Design review of the part shown in the three views and the two pictorial views. Dimensions are in mm from the part's minimum x, y and z. A direction names the side the tool comes from. Round coordinates to 2 decimals unless told otherwise and drop trailing zeros. Order: outer loops, then holes, each group sorted by start corner. A loop starts at its lowest first (then second) coordinate and runs counter-clockwise, first axis right, second up.
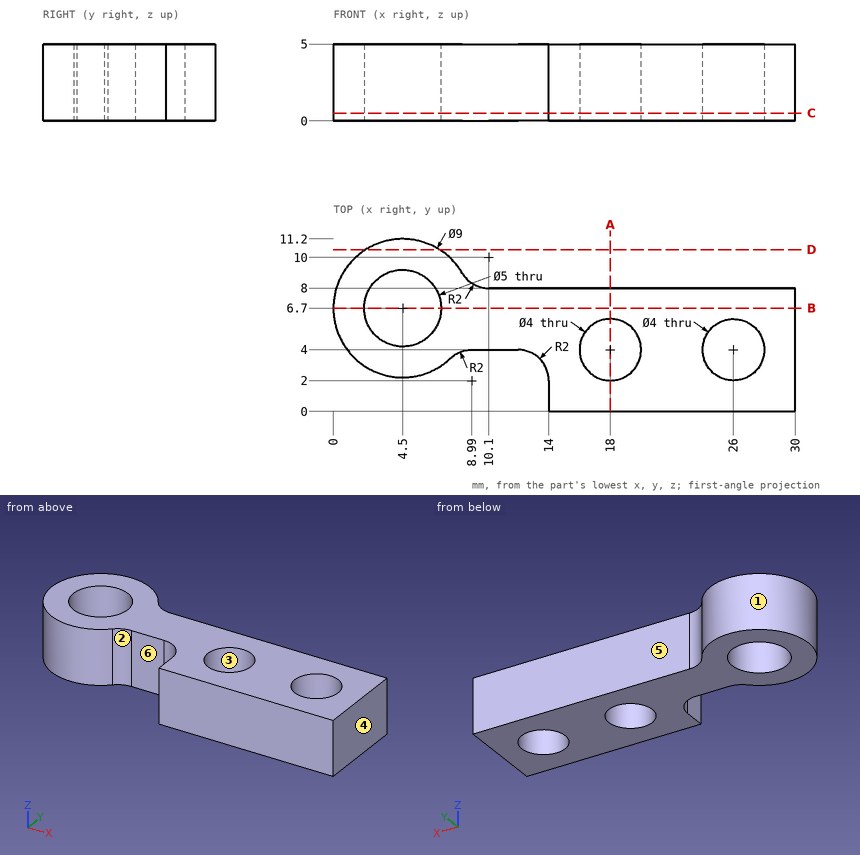
(1) Consider section A-A (x = 18). Write out the cut boundary in (y, z).
Data:
outline: (0, 0) - (2, 0) - (2, 5) - (0, 5) - close; (6, 0) - (8, 0) - (8, 5) - (6, 5) - close
(2) Insertion check: pin 1 (2.5 mm diameter, centred on x = 10, z = 2.5, fed in from -Y); pin 2 (0.6 mm diameter, centred on y = 0.5, z = 3.5, fed in from -X); pin 3 (5 mm diameter, centred on x = 26, y = 4, fed in from +Z); pin 4 (2 mm diameter, centred on y = 10, z = 1, fed in from +X). Each pin has a flat end and moves straight along its axis. Give the tip position at first contact, or say it passes through.
Data:
pin 1: stops at y = 3.99
pin 2: stops at x = 14
pin 3: stops at z = 5
pin 4: stops at x = 8.37
(3) Consider section C-C (z = 0.5). Write out the cut boundary in (x, y).
Data:
outline: (7.61, 3.45) arc R2 cw to (8.99, 4) - (12, 4) arc R2 cw to (14, 2) - (14, 0) - (30, 0) - (30, 8) - (10.1, 8) arc R2 cw to (8.38, 8.98) arc R4.5 ccw (long way) to start; hole circle Ø5 at (4.5, 6.7); hole circle Ø4 at (18, 4); hole circle Ø4 at (26, 4)
(4) For the marked faces 4, 5 and 6, list the 3-axis set-ups (+Z, -Z, +X, -X, +Y, -Y) from which the entire face can be reached by the end or side of a thin tool; tool diameter is ignored.
Data:
face 4: +Z, -Z, +X, +Y, -Y
face 5: +Z, -Z, +X, +Y
face 6: +Z, -Z, -Y
(5) Consider section D-D (y = 10.5). Write out the cut boundary in (x, z), and give its area (3 significant figures).
Data:
outline: (2.09, 0) - (6.91, 0) - (6.91, 5) - (2.09, 5) - close
area: 24.1 mm2
(6) Draft analysis for pull direction Y (two halves, no side actions). For the marked faces 1, 2 and 3, state which applies: pulls with the +Y half, pulls with the -Y half, needs draft (parallel to the pull), parting line crosses it, or undercut.
Data:
face 1: parting line crosses it
face 2: pulls with the -Y half
face 3: undercut
(7) Consider section B-B (y = 6.7). Write out the cut boundary in (x, z).
Data:
outline: (0, 0) - (2, 0) - (2, 5) - (0, 5) - close; (7, 0) - (30, 0) - (30, 5) - (7, 5) - close
(8) To check wall thickness, follow probe 1 along X at (y, z) = (5.5, 2.15); probe 2 along Y at (x, z) = (26, 2.5); probe 3 along X at (y, z) = (1.25, 1.3). State the ranges of each line that lie inside material, in increasing order.
Data:
probe 1: x = 0.16 to 2.31, 6.69 to 16.68, 19.32 to 24.68, 27.32 to 30
probe 2: y = 0 to 2, 6 to 8
probe 3: x = 14 to 30
